from build123d import *

# Parameters (mm, degrees)
F0_W     = 194.9958
F0_H     = 84.9884
F1_DEPTH = 1.5875
F2_W     = 179.3494
F2_H     = 69.3452
F2_W_2   = 64.45
F2_H_2   = 11.61
F3_DEPTH = 2.54
F4_R     = 2.45
F5_DEPTH = 22.86
F6_W     = 11.75
F6_H     = 11.75
F7_DEPTH = 25.4
F8_T     = -2.54


with BuildPart() as f1:
    # F0 (on Top) → F1 (new body)
    with BuildSketch(Plane.XY):
        Rectangle(F0_W, F0_H)
    extrude(amount=F1_DEPTH)

    # F2 (on face) → F3 (join)
    with BuildSketch(Plane.XY.offset(1.5875)):
        with Locations((0, 0.0016)):
            Rectangle(F2_W, F2_H)
        with Locations((-49.5541132987, 20.0935862262)):
            Rectangle(F2_W_2, F2_H_2, mode=Mode.SUBTRACT)
        with Locations((-49.5541132987, 20.0935862262)):
            Rectangle(F2_W_2, F2_H_2)
    extrude(amount=F3_DEPTH)

    # F4 (on face) → F5 (cut)
    with BuildSketch(Plane(origin=(0, 0, 0), x_dir=(1, 0, 0), z_dir=(0, 0, -1))):
        with Locations((-38.0999999963, 17.779997108)):
            Circle(F4_R)
        with Locations((45.2885175493, 17.780080176)):
            Circle(F4_R)
        with Locations((21.3446233022, 17.7799198239)):
            Circle(F4_R)
        with Locations((-14.1500980391, 17.780002892)):
            Circle(F4_R)
    extrude(amount=-F5_DEPTH, mode=Mode.SUBTRACT)

    # F6 (on face) → F7 (cut)
    with BuildSketch(Plane.XY.offset(4.1275)):
        with Locations((45.4056928721, 12.6071161675)):
            Rectangle(F6_W, F6_H)
        with Locations((21.3366928721, 12.610067341)):
            Rectangle(F6_W, F6_H)
        with Locations((-16.5584006092, 12.610067341)):
            Rectangle(F6_W, F6_H)
        with Locations((-40.6274006092, 12.610067341)):
            Rectangle(F6_W, F6_H)
    extrude(amount=-F7_DEPTH, mode=Mode.SUBTRACT)

    # F8
    f8_openings = [f1.faces().sort_by_distance(p)[0] for p in [
        (-0.134693, -0.47441, 4.1275),
    ]]
    offset(amount=F8_T, openings=f8_openings, kind=Kind.INTERSECTION)


solid = f1.part
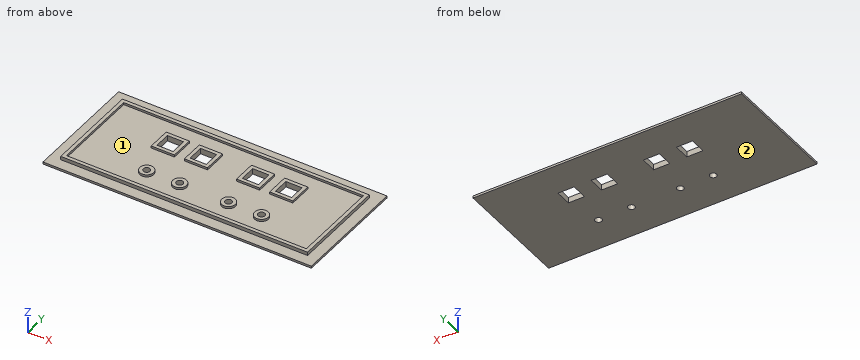
For this review, take the finished solid that the model builds, in its own axes (mm). Face numbers are marked on the shaded views. Coordinates: 2 decimals unless noted, no trailing zeros. Loops run counter-clockwise (first coordinate to the right, second up) from the corner with the lowest first, then second, coordinate; pieces in that order, holes last. Notation, with made-up numbers: (-2, 23) - (8, 23) arc R16 ccw to (8, 27) - close; hole circle Ø6 at (33.25, 46.25). An arc over 180 degrees is marked (long way). Use a Markdown table: item, result. Add a question column.
Item 1: We need section B-B (x = 56.5). Give the boundary of the cut face in (y, z).
Item 2: We need section A-A (x = -38.1). Give the boundary of the cut face in (y, z), and give its area (3 significant figures).
Item 3: For line 1 (X direction, y = 15, z = 0.9); line 2 (Y direction, x = -14, z = 2.8); line 3 (Y direction, x = -38.1, z = 1.7), list the stretches that pass through material, from the lowest coordinate up.
Item 4: We need section D-D (x = 21). Give the boundary of the cut face in (y, z), and give its area (3 significant figures).
Item 5: Insertion check: pin 1 Ø1.2 at (x, z) = (-42, 3) entering from -Y; pin 2 Ø0.5 at (x, z) = (-12.5, 3) entering from +Y; pin 3 Ø1.5 at (x, y) = (-58, -7.5) entering from +Z. Each pin has a flat end and moves straight along its axis. Give the tip position at first contact, or say it passes through.
Item 6: We need section C-C (y = 11). Give the number of separate pieces and of enclosed holes in the cut face, and give its area (3 significant figures).
Item 7: Mouldability with a two-part tool opening along Y and no side actions: class the marked faces 1 and 2 as pulls with the +Y half, pulls with the -Y half, needs draft (parallel to the pull), parting line crosses it, or undercut.
Results list:
| question | item | result |
|---|---|---|
| 1 | outline | (-42.49, 0) - (42.49, 0) - (42.49, 1.59) - (34.67, 1.59) - (34.67, 4.13) - (32.13, 4.13) - (32.13, 2.54) - (-32.13, 2.54) - (-32.13, 4.13) - (-34.67, 4.13) - (-34.67, 1.59) - (-42.49, 1.59) - close |
| 2 | outline | (-42.49, 0) - (-20.23, 0) - (-20.23, 4.13) - (-22.77, 4.13) - (-22.77, 2.54) - (-32.13, 2.54) - (-32.13, 4.13) - (-34.67, 4.13) - (-34.67, 1.59) - (-42.49, 1.59) - close; (-15.33, 0) - (6.74, 0) - (6.74, 4.13) - (4.2, 4.13) - (4.2, 2.54) - (-12.79, 2.54) - (-12.79, 4.13) - (-15.33, 4.13) - close; (18.49, 0) - (42.49, 0) - (42.49, 1.59) - (34.67, 1.59) - (34.67, 4.13) - (32.13, 4.13) - (32.13, 2.54) - (21.03, 2.54) - (21.03, 4.13) - (18.49, 4.13) - close |
| 2 | area | 183 mm^2 |
| 3 | line 1 | x = -97.5 to -46.5, -34.75 to -22.43, -10.68 to 15.46, 27.21 to 39.53, 51.28 to 97.5 |
| 3 | line 2 | y = -34.67 to -32.13, -22.77 to -20.23, -15.33 to -12.79, 4.2 to 6.74, 18.49 to 21.03, 32.13 to 34.67 |
| 3 | line 3 | y = -34.67 to -20.23, -15.33 to 6.74, 18.49 to 34.67 |
| 4 | outline | (-42.49, 0) - (-20.21, 0) - (-20.21, 4.13) - (-22.76, 4.13) - (-22.76, 2.54) - (-32.13, 2.54) - (-32.13, 4.13) - (-34.67, 4.13) - (-34.67, 1.59) - (-42.49, 1.59) - close; (-15.35, 0) - (6.74, 0) - (6.74, 4.13) - (4.2, 4.13) - (4.2, 2.54) - (-12.8, 2.54) - (-12.8, 4.13) - (-15.35, 4.13) - close; (18.49, 0) - (42.49, 0) - (42.49, 1.59) - (34.67, 1.59) - (34.67, 4.13) - (32.13, 4.13) - (32.13, 2.54) - (21.03, 2.54) - (21.03, 4.13) - (18.49, 4.13) - close |
| 4 | area | 183 mm^2 |
| 5 | pin 1 | stops at y = -34.67 |
| 5 | pin 2 | stops at y = 34.67 |
| 5 | pin 3 | stops at z = 2.54 |
| 6 | separate pieces | 5 |
| 6 | enclosed holes | 0 |
| 6 | area | 401 mm^2 |
| 7 | face 1 | undercut |
| 7 | face 2 | needs draft |
